Design review of the part built by this model. Coordinates are the model's own, in mm. Give positions to 0.01 mm unless a question says otherwise; leave off trailing zeros. Order: outer loops, then holes, each group sorted by start corner. A loop starts at its lowest first (then second) coordinate and runs counter-clockwise, first axis right, second up. Notation, with made-up numbers: (17.5, 75.5) - (65.5, 75.5) arc R17 cw to (65.5, 105.5) - close; hole circle Ø11 at (54, 88). An arc over 180 degrees is marked (long way). Write each question's results on one line, items separated by ' | '. Start each with the question number.
```python
from build123d import *

# Parameters (mm, degrees)
SKETCH1_R            = 25.4
BOSS_EXTRUDE1_DEPTH  = 31.75
SKETCH2_R            = 16
CUT_EXTRUDE1_DEPTH   = 0.25
M4_CLEARANCE_HOLE1_D = 4.5
SKETCH6_R            = 5
CUT_EXTRUDE2_DEPTH   = 48.77624933
BOSS_EXTRUDE2_DEPTH  = 31.8


with BuildPart() as part:
    # Sketch1 → Boss-Extrude1 (new body)
    with BuildSketch(Plane.XY):
        Circle(SKETCH1_R)
    extrude(amount=-BOSS_EXTRUDE1_DEPTH)

    # Sketch2 → Cut-Extrude1 (cut)
    with BuildSketch(Plane.XY):
        Circle(SKETCH2_R)
    extrude(amount=-CUT_EXTRUDE1_DEPTH, mode=Mode.SUBTRACT)

    # M4 Clearance Hole1 (through all)
    with Locations(Plane.XY.offset(-0.25)):
        with Locations((-8.838834765, 8.838834765), (8.838834765, 8.838834765), (-8.838834765, -8.838834765), (8.838834765, -8.838834765)):
            Hole(M4_CLEARANCE_HOLE1_D / 2)

    # Sketch6 → Cut-Extrude2 (cut, through all)
    with BuildSketch(Plane.XY.offset(-0.25)):
        Circle(SKETCH6_R)
    extrude(amount=-CUT_EXTRUDE2_DEPTH, mode=Mode.SUBTRACT)

    # Sketch8 → Boss-Extrude2 (add)
    with BuildSketch(Plane.XY):
        with BuildLine():
            Line((6.796221999, -24.473891528), (16.535857352, -34.213526881))
            ThreePointArc((16.535857352, -34.213526881), (26.870057685, -26.870057685), (34.213526881, -16.535857352))
            Line((34.213526881, -16.535857352), (24.473891528, -6.796221999))
            ThreePointArc((24.473891528, -6.796221999), (17.960512242, -17.960512242), (6.796221999, -24.473891528))
        make_face()
    extrude(amount=-BOSS_EXTRUDE2_DEPTH)


solid = part.part
```
Q1. Insertion check: pin 1 Ø12 at (x, z) = (24, -4.5) entering from -Y; pin 2 Ø6 at (x, z) = (24.5, -10.5) entering from +Y; pin 3 Ø10 at (x, z) = (-15.5, -25) entering from +Y. Each pin has a flat end and moves straight along its axis. Give the tip position at first contact, or say it passes through.
Q2. Add section C-C (z = -23.5). Give the boundary of the cut face in (x, y), plus the area to 3 significant figures.
Q3. For line 1 (Y direction, x = 0, z = -0.05); line 2 (Y direction, x = 0, z = -24); line 3 (X direction, y = 10, z = -10), list the stretches that pass through material, from the lowest coordinate up. Write a range as [from, to].
Q4. Add section D-D (y = -8). Give the boundary of the cut face in (x, z), plus the area to 3 significant figures.
Q5. Draft analysis for pull direction X (two halves, no side actions). For faces 1 (the flat face through (-4, 4, -0.25)), 2 (the flat face through (29.41, -11.73, -15.68)), 3 (the flat face through (23, -23, -31.8)), state which applies: pulls with the +X half, pulls with the -X half, needs draft (parallel to the pull), parting line crosses it, or undercut.
Q6. Add section A-A (x = 0). Give the boundary of the cut face in (y, z), plus the area to 3 significant figures.
Verdict:
1) pin 1: stops at y = -33.47 | pin 2: stops at y = 13.52 | pin 3: stops at y = 23.13
2) outline: (6.8, -24.47) - (16.54, -34.21) arc R38 ccw to (34.21, -16.54) - (24.47, -6.8) arc R25.4 ccw (long way) to start; hole circle Ø4.5 at (-8.84, -8.84); hole circle Ø4.5 at (-8.84, 8.84); hole circle Ø10 at (0, 0); hole circle Ø4.5 at (8.84, -8.84); hole circle Ø4.5 at (8.84, 8.84) | area: 2,210 mm2
3) line 1: y = [-25.4, -16], [16, 25.4] | line 2: y = [-25.4, -5], [5, 25.4] | line 3: x = [-23.35, -10.77], [-6.91, 6.91], [10.77, 23.35]
4) outline: (-24.11, -31.75) - (-10.93, -31.75) - (-10.93, -0.25) - (-13.86, -0.25) - (-13.86, 0) - (-24.11, 0) - close; (-6.75, -31.75) - (6.75, -31.75) - (6.75, -0.25) - (-6.75, -0.25) - close; (10.93, -31.75) - (24.11, -31.75) - (24.11, -31.8) - (25.68, -31.8) - (25.68, 0) - (13.86, 0) - (13.86, -0.25) - (10.93, -0.25) - close | area: 1,310 mm2
5) face 1: undercut | face 2: pulls with the +X half | face 3: needs draft
6) outline: (-25.4, -31.75) - (-5, -31.75) - (-5, -0.25) - (-16, -0.25) - (-16, 0) - (-25.4, 0) - close; (5, -31.75) - (25.4, -31.75) - (25.4, 0) - (16, 0) - (16, -0.25) - (5, -0.25) - close | area: 1,290 mm2
